Verification items for the finished model (mm, model axes). A direction names the side the tool comes from. Round coordinates to 2 decimals unless told otherwise and drop trailing zeros. Order: outer loops, then holes, each group sorted by start corner. A loop starts at its lowest first (then second) coordinate and runs counter-clockwise, first axis right, second up.
Autodesk Inventor part; units mm, degrees
ref_plane "YZ Plane" through (0, 0, 0) normal (1, 0, 0) x (0, 1, 0)
ref_plane "XZ Plane" through (0, 0, 0) normal (0, 1, 0) x (-1, 0, 0)
ref_plane "XY Plane" through (0, 0, 0) normal (0, 0, 1) x (1, 0, 0)
sketch "Sketch1" plane through (0, 0, 0) normal (0, 0, 1) x (1, 0, 0)
  line L0 (0, 0) -> (23.114, 0)
  line L1 (23.114, 0) -> (23.114, 15.0368)
  line L2 (23.114, 15.0368) -> (0, 15.0368)
  line L3 (0, 15.0368) -> (0, 0)
  dimension "d0" = 15.0368
  dimension "d1" = 23.114
extrude "Extrusion1" add sketch "Sketch1" along normal blind 11.7348
sketch "Sketch2" plane through (0, 0, 11.7348) normal (0, 0, 1) x (1, 0, 0)
  line L0 (23.114, 0) -> (23.114, 3.6138)
  line L1 (23.114, 0) -> (23.114, 15.0368)
  line L2 (0, 0) -> (23.114, 0)
  line L3 (20.3034, 0) -> (23.114, 0)
  line L4 (23.114, 3.6138) -> (20.3034, 0)
extrude "Extrusion2" cut sketch "Sketch2" against normal blind 11.7348
sketch "Sketch3" plane through (0, 0, 11.7348) normal (0, 0, 1) x (1, 0, 0)
  line L0 (-4.6433, 16.5606) -> (27.1067, 16.5606)
  line L1 (27.1067, 16.5606) -> (27.1067, 15.0366)
  line L2 (27.1067, 15.0366) -> (-4.6433, 15.0366)
  line L3 (-4.6433, 15.0366) -> (-4.6433, 16.5606)
  line L4 (23.114, 15.0368) -> (0, 15.0368)
  point P0 (0, 0)
  dimension "d6" = 31.75
  dimension "d7" = 1.524
extrude "Extrusion3" add sketch "Sketch3" against normal blind 11.7348
sketch "Sketch4" plane through (0, 0, 11.7348) normal (0, 0, 1) x (1, 0, 0)
  line L0 (-4.6433, 16.5606) -> (27.1067, 16.5606)
  line L1 (0, 16.5606) -> (23.1157, 16.5606)
  line L2 (23.1157, 16.5606) -> (23.1157, 21.3866)
  line L3 (23.1157, 21.3866) -> (0, 21.3866)
  line L4 (0, 21.3866) -> (0, 16.5606)
  point P0 (0, 0)
  dimension "d10" = 4.826
extrude "Extrusion4" add sketch "Sketch4" against normal up to surface (11.7348 mm away)
sketch "Sketch5" plane through (0, 21.3866, 11.7348) normal (0, 1, 0) x (1, 0, 0)
  circle A0 centre (16.764, 5.8674) radius 4.8959
  line L0 (0, 11.7348) -> (23.1157, 11.7348)
  line L1 (0, 0) -> (0, 11.7348)
  line L2 (23.1157, 0) -> (0, 0)
  line L3 (23.1157, 0) -> (23.1157, 11.7348)
  point P0 (0, 11.7348)
  dimension "d14" = 9.7917
  dimension "d39" = 11.7348
  dimension "d40" = 5.8674
  dimension "d46" = 16.764
extrude "Extrusion5" add sketch "Sketch5" along normal blind 3.81 contours A0
sketch "Sketch6" plane through (16.764, 25.1966, 5.8674) normal (0, 1, 0) x (1, 0, 0)
  circle A0 centre (0, 0) radius 4.8958
  arc A1 (-4.5107, 1.9034) -> (-5.2123, 0) centre (-4.8064, 0.9314) ccw
  line L0 (-5.2123, 0) -> (-5.7995, 0)
  line L1 (-5.7995, 0) -> (-5.7995, -3.5655)
  line L2 (-5.7995, -3.5655) -> (-3.355, -3.5655)
  line L3 (-4.228, 0.0962) -> (-4.228, 0.1127)
  point P0 (-16.764, 5.8674)
  point P1 (-5.5059, 0)
  dimension "d35" = 2.4445
  dimension "d36" = 3.5655
  dimension "d37" = 1.016
  dimension "d38" = 0.9314
extrude "Extrusion6" add sketch "Sketch6" against normal blind 3.9878 contours A0 L2 L1 L0 A1
sketch "Sketch7" plane through (0, 25.1966, 11.7348) normal (0, 1, 0) x (1, 0, 0)
  circle A0 centre (16.9713, 5.8977) radius 1.7145
  point P0 (0, 11.7348)
  dimension "d19" = 3.429
extrude "Extrusion7" add sketch "Sketch7" along normal blind 6.35
sketch "Sketch8" plane through (16.9713, 31.5466, 5.8371) normal (0, 1, 0) x (1, 0, 0)
  circle A0 centre (0, 0) radius 0.41
  point P0 (-16.9713, 5.8371)
extrude "Extrusion8" cut sketch "Sketch8" against normal blind 0.254
sketch "Sketch9" plane through (-4.6433, 16.5606, 11.7348) normal (0, 1, 0) x (1, 0, 0)
  line L0 (4.6433, 0) -> (4.6433, 11.7348)
  line L1 (0, 0) -> (0, 11.7348)
  line L2 (31.75, 0) -> (31.75, 11.7348)
  line L3 (27.759, 0) -> (27.759, 11.7348)
  circle A0 centre (2.3241, 5.8674) radius 1.524
  line L4 (0, 0) -> (4.6433, 0)
  circle A1 centre (29.7561, 5.8674) radius 1.524
  line L5 (27.759, 11.7348) -> (31.75, 11.7348)
  dimension "d24" = 4.6433
  dimension "d25" = 3.991
  dimension "d26" = 3.048
  dimension "d27" = 2.3241
  dimension "d28" = 11.7348
  dimension "d29" = 5.8674
  dimension "d30" = 3.048
  dimension "d31" = 5.8674
  dimension "d32" = 1.9939
extrude "Extrusion9" cut sketch "Sketch9" against normal blind 25.4
sketch "Sketch11" plane through (-4.6433, 16.5606, 11.7348) normal (0, 1, 0) x (1, 0, 0)
  circle A0 centre (29.7561, 5.8674) radius 1.524
  circle A1 centre (29.7561, 5.8674) radius 1.524
  line L0 (27.759, 11.7348) -> (27.759, 0)
  line L1 (27.759, 0) -> (31.75, 0)
  line L2 (31.75, 0) -> (31.75, 11.7348)
  line L3 (27.759, 11.7348) -> (31.75, 11.7348)
  point P0 (4.6433, 11.7348)
extrude "Extrusion10" cut sketch "Sketch11" against normal blind 25.4
1) Sectioned sample at A-A on x = -1.75. Record the cut outline in (y, z), then the cut area to 3 significant figures.
2) Go/stop test with flat-tipped pins: pin 1 Ø1.2 at (x, y) = (12, 24) entering from +Z; pin 2 Ø5 at (x, z) = (-1.5, 4.5) entering from +Y; pin 3 Ø1.5 at (x, y) = (10, 25) entering from +Z; pin 4 Ø2 at (x, z) = (10, 5) entering from +Y. Record where each tip stops, or that it passes through.
3) Sectioned sample at D-D on x = 17.75. Record the cut outline in (y, z), then the cut area to 3 significant figures.
4) Sectioned sample at B-B on y = 16. Record the cut outline in (x, z).
5) Tool access check on faces 1 (the flat face through (12, 23, 9.433)), 2 (the flat face through (0, 8, 6)), 3 (the flat face through (-4, 16.561, 6)), 4 (the cylindrical face through (15.26, 28.33, 5.91)). Record the directions out of +Z, -Z, +X, -X, +Y, -Y that give a thin tool (end or side, any length) a straight path to the whole face; none if there is none.
6) Scan lines: probe 1 along Y at (x, z) = (6.5, 10.75); probe 2 along X at (y, z) = (14.5, 3.75); probe 3 along Y at (x, z) = (12, 8.25). Record each from-to range of solid material in increasing order.
Returned:
1. outline: (15.04, 0) - (16.56, 0) - (16.56, 4.45) - (15.04, 4.45) - close; (15.04, 7.28) - (16.56, 7.28) - (16.56, 11.73) - (15.04, 11.73) - close
1. area: 13.6 mm2
2. pin 1: stops at z = 9.43
2. pin 2: stops at y = 21.39
2. pin 3: passes through
2. pin 4: stops at y = 25.2
3. outline: (0, 0) - (21.39, 0) - (21.39, 1.07) - (25.2, 1.07) - (25.2, 4.31) - (31.55, 4.31) - (31.55, 7.36) - (25.2, 7.36) - (25.2, 10.66) - (21.39, 10.66) - (21.39, 11.73) - (0, 11.73) - close
3. area: 307 mm2
4. outline: (-4.64, 0) - (23.12, 0) - (23.12, 11.73) - (-4.64, 11.73) - close; hole circle Ø3.05 at (-2.32, 5.87)
5. face 1: +Z, -X, +Y
5. face 2: +Z, -Z, -X, -Y
5. face 3: +Z, -Z, -X, +Y
5. face 4: +Y
6. probe 1: y = 0 to 21.39
6. probe 2: x = 0 to 23.11
6. probe 3: y = 0 to 25.2
